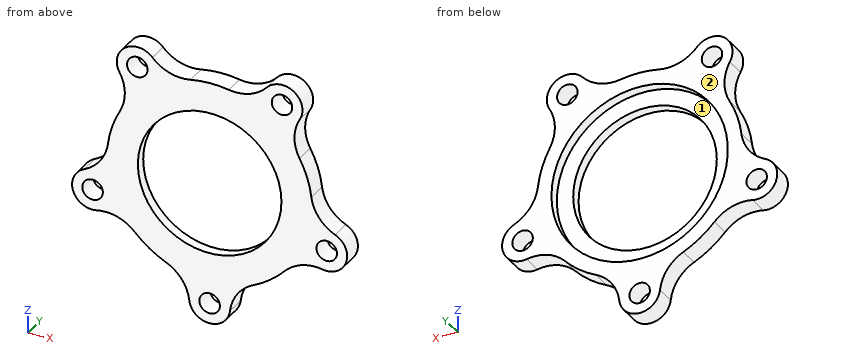
```python
from build123d import *

# Parameters (mm, degrees)
SKETCH1_R           = 3.175
SKETCH1_R_2         = 27.305
BOSS_EXTRUDE4_DEPTH = 6.35
SKETCH1_6_R         = 27.305
SKETCH1_6_R_2       = 22.225
BOSS_EXTRUDE5_DEPTH = 3.175
FILLET2_R           = 12.7


with BuildPart() as part:
    # Sketch1 → Boss-Extrude4 (new body)
    with BuildSketch(Plane(origin=(0, 0, 0), x_dir=(1, 0, 0), z_dir=(0, 1, 0))):
        with BuildLine():
            Line((6.35, 31.108519733), (6.35, 38.1))
            ThreePointArc((6.35, 38.1), (0, 44.45), (-6.35, 38.1))
            Line((-6.35, 38.1), (-6.35, 31.108519733))
            ThreePointArc((-6.35, 31.108519733), (-18.66218176, 25.686289571), (-27.62370249, 15.652270146))
            Line((-27.62370249, 15.652270146), (-34.272995357, 17.812756364))
            ThreePointArc((-34.272995357, 17.812756364), (-42.274462149, 13.7358054), (-38.197511185, 5.734338607))
            Line((-38.197511185, 5.734338607), (-31.548218319, 3.573852389))
            ThreePointArc((-31.548218319, 3.573852389), (-30.196044392, -9.811289571), (-23.422387034, -21.434884782))
            Line((-23.422387034, -21.434884782), (-27.531876027, -27.091111134))
            ThreePointArc((-27.531876027, -27.091111134), (-26.127054464, -35.9608054), (-17.257360198, -34.555983838))
            Line((-17.257360198, -34.555983838), (-13.147871206, -28.899757486))
            ThreePointArc((-13.147871206, -28.899757486), (0, -31.75), (13.147871206, -28.899757486))
            Line((13.147871206, -28.899757486), (17.257360198, -34.555983838))
            ThreePointArc((17.257360198, -34.555983838), (26.127054464, -35.9608054), (27.531876027, -27.091111134))
            Line((27.531876027, -27.091111134), (23.422387034, -21.434884782))
            ThreePointArc((23.422387034, -21.434884782), (30.196044392, -9.811289571), (31.548218319, 3.573852389))
            Line((31.548218319, 3.573852389), (38.197511185, 5.734338607))
            ThreePointArc((38.197511185, 5.734338607), (42.274462149, 13.7358054), (34.272995357, 17.812756364))
            Line((34.272995357, 17.812756364), (27.62370249, 15.652270146))
            ThreePointArc((27.62370249, 15.652270146), (18.66218176, 25.686289571), (6.35, 31.108519733))
        make_face()
        with Locations((0, 38.1)):
            Circle(SKETCH1_R, mode=Mode.SUBTRACT)
        Circle(SKETCH1_R_2, mode=Mode.SUBTRACT)
        with Locations((36.235253271, 11.773547486)):
            Circle(SKETCH1_R, mode=Mode.SUBTRACT)
        with Locations((-36.235253271, 11.773547486)):
            Circle(SKETCH1_R, mode=Mode.SUBTRACT)
        with Locations((22.394618112, -30.823547486)):
            Circle(SKETCH1_R, mode=Mode.SUBTRACT)
        with Locations((-22.394618112, -30.823547486)):
            Circle(SKETCH1_R, mode=Mode.SUBTRACT)
    extrude(amount=BOSS_EXTRUDE4_DEPTH)

    # Sketch1<6> → Boss-Extrude5 (add)
    with BuildSketch(Plane(origin=(0, 0, 0), x_dir=(1, 0, 0), z_dir=(0, 1, 0))):
        Circle(SKETCH1_6_R)
        Circle(SKETCH1_6_R_2, mode=Mode.SUBTRACT)
    extrude(amount=BOSS_EXTRUDE5_DEPTH)

    # Fillet2
    fillet2_edges = [part.edges().sort_by_distance(p)[0] for p in [
        (27.62370249, 3.175, -15.652270146),
        (31.548218319, 3.175, -3.573852389),
        (23.422387034, 3.175, 21.434884782),
        (13.147871206, 3.175, 28.899757486),
        (-13.147871206, 3.175, 28.899757486),
        (-23.422387034, 3.175, 21.434884782),
        (-31.548218319, 3.175, -3.573852389),
        (-27.62370249, 3.175, -15.652270146),
        (-6.35, 3.175, -31.108519733),
        (6.35, 3.175, -31.108519733),
    ]]
    fillet(fillet2_edges, radius=FILLET2_R)


solid = part.part
```
Can you work these out from the model? Positions are in its coordinate system, mm. Face numbers are marked on the shaded views. Round coordinates to 2 decimals unless told otherwise and drop trailing zeros. Loops run counter-clockwise (first coordinate to the right, second up) from the corner with the lowest first, then second, coordinate; pieces in that order, holes last. Notation, with made-up numbers: M -1.5,-17.75 L 44.5,-17.75 A20 cw 44.5,-4.75 Z; hole C 10,8.5 d7. An arc over 180 degrees is marked long. Answer as a JSON object with one key per item and string values. Group by question number.
Q1. Will these pins go through, and if not, where does the flat tip stop? pin 1 (5 mm diameter, centred on x = -36.24, z = -11.77, fed in from +Y); pin 2 (3 mm diameter, centred on y = 1, z = -23.5, fed in from +X); pin 3 (1 mm diameter, centred on y = 2, z = -36, fed in from +X); pin 4 (1.5 mm diameter, centred on y = 1.5, z = -23, fed in from -X).
Q2. Imagine slicing it at A-A, the plane x = 0. Please give me the cut outline in (y, z) (3 decimals), then the cut area to 3 significant figures.
Q3. Please list where these lines run through material, in increasing order: L1, parallel to Z at x = 0, y = 3.95 (3 decimals); L2, parallel to X at y = 2.5, z = 33; L3, parallel to Z at x = -20, y = 4.5.
Q4. Imagine slicing it at C-C, the plane z = 11.5. Please give me the cut outline in (x, y) (3 decimals), then the cut area to 3 significant figures.
Q5. Imagine slicing it at B-B, the plane z = -14. Please give me the cut outline in (x, y) (3 decimals).
Q6. Imagine slicing it at D-D, the plane y = 4.75. Count the separate pieces of the cut face and the enclosed holes in it, then the cut area to 3 significant figures.
Q7. We'd pull the mould along X, two halves only. Please class the marked faces 1 and 2: +X half, -X half, draft (parallel to the pull), parting line (faces both ways), or undercut.
Findings:
{
 "1": {"pin 1": "passes through", "pin 2": "stops at x = 22.89", "pin 3": "stops at x = 7.14", "pin 4": "stops at x = -22.65"},
 "2": {"outline": "M 0,-44.45 L 6.35,-44.45 L 6.35,-41.275 L 0,-41.275 Z; M 0,-34.925 L 6.35,-34.925 L 6.35,-27.305 L 3.175,-27.305 L 3.175,-22.225 L 0,-22.225 Z; M 0,22.225 L 3.175,22.225 L 3.175,27.305 L 6.35,27.305 L 6.35,31.75 L 0,31.75 Z", "area": "129 mm2"},
 "3": {"L1": "z = -44.45 to -41.275, -34.925 to -27.305, 27.305 to 31.75", "L2": "x = -28.36 to -24.71, -20.08 to -15.22, 15.22 to 20.08, 24.71 to 28.36", "L3": "z = -24.66 to -18.59, 18.59 to 28.74, 32.91 to 36.7"},
 "4": {"outline": "M -29.594,0 L -19.018,0 L -19.018,3.175 L -24.765,3.175 L -24.765,6.35 L -29.594,6.35 Z; M 19.018,0 L 29.594,0 L 29.594,6.35 L 24.765,6.35 L 24.765,3.175 L 19.018,3.175 Z", "area": "97.8 mm2"},
 "5": {"outline": "M -42.182,0 L -38.499,0 L -38.499,6.35 L -42.182,6.35 Z; M -33.972,0 L -17.261,0 L -17.261,3.175 L -23.443,3.175 L -23.443,6.35 L -33.972,6.35 Z; M 17.261,0 L 33.972,0 L 33.972,6.35 L 23.443,6.35 L 23.443,3.175 L 17.261,3.175 Z; M 38.499,0 L 42.182,0 L 42.182,6.35 L 38.499,6.35 Z"},
 "6": {"separate pieces": "1", "enclosed holes": "6", "area": "1,530 mm2"},
 "7": {"face 1": "undercut", "face 2": "draft"}
}
